Check sheet for the modelled part. Datum: model origin and axes. Units: mm. Round coordinates to 2 decimals unless told otherwise and drop trailing zeros. Order: outer loops, then holes, each group sorted by start corner. A loop starts at its lowest first (then second) coordinate and runs counter-clockwise, first axis right, second up. Notation, with made-up numbers: (64, 84) -> (80, 84) arc R22 ccw to (80, 90) -> close; hole circle Ø7 at (-40, 15.25). An arc over 180 degrees is marked (long way). Answer in a Markdown table with one row per item.
```python
from build123d import *

# Parameters (mm, degrees)
SKETCH_2_R          = 1.5
EXTRUDE_1_DEPTH     = 10
CUT_EXTRUDE_START   = -7.5
SKETCH_3_R          = 1.5
SKETCH_3_R_2        = 1.2
CUT_EXTRUDE_1_DEPTH = 0.6
CHAMFER_1_SIZE      = 0.2


with BuildPart() as part:
    # 草图2 → 凸台-拉伸1 (new body, symmetric)
    with BuildSketch(Plane(origin=(0, 0, 0), x_dir=(0, 0, -1), z_dir=(1, 0, 0))):
        Circle(SKETCH_2_R)
    extrude(amount=EXTRUDE_1_DEPTH, both=True)

    # 草图3 → 切除-拉伸1 (cut)
    with BuildSketch(Plane(origin=(0, 0, 0), x_dir=(0, 0, -1), z_dir=(1, 0, 0)).offset(CUT_EXTRUDE_START)):
        Circle(SKETCH_3_R)
        Circle(SKETCH_3_R_2, mode=Mode.SUBTRACT)
    cut_extrude_1 = extrude(amount=-CUT_EXTRUDE_1_DEPTH, mode=Mode.SUBTRACT)

    # 镜向1: 切除-拉伸1 across plane
    add(cut_extrude_1.mirror(Plane(origin=(0, 0, 0), x_dir=(0, 0, 1), z_dir=(1, 0, 0))), mode=Mode.SUBTRACT)

    # 倒角1
    chamfer_1_edges = [part.edges().sort_by_distance(p)[0] for p in [
        (-10, 0, 1.5),
        (10, 0, 1.5),
    ]]
    chamfer(chamfer_1_edges, length=CHAMFER_1_SIZE)


solid = part.part
```
(1) Section check A-A on x = -2. Record the boundary of the cut face in (y, z), plus the area to 3 significant figures.
Solutions:
| item | result |
|---|---|
| outline | circle Ø3 at (0, 0) |
| area | 7.07 mm^2 |
(2) Scan lines: probe 1 along X at (y, z) = (0.9, 0.85); probe 2 along Z at (x, y) = (5, -0.1); probe 3 along Z at (x, y) = (6.75, 0.9). Record each from-to range of solid material in increasing order. Write a range as from..to.
Solutions:
| item | result |
|---|---|
| probe 1 | -10..-8.1, -7.5..7.5, 8.1..10 |
| probe 2 | -1.5..1.5 |
| probe 3 | -1.2..1.2 |
(3) Draft check along X on faces 1 (the cylindrical face through (-7.8, 1.01, -0.65)), 2 (the flat face through (10, 0, 0)), 3 (the cylindrical face through (7.8, 1.01, -0.65)), 4 (the cylindrical face through (8.96, 0.07, 1.5)). Enter one of: pulls with the +X half, pulls with the -X half, needs draft (parallel to the pull), parting line crosses it, or undercut.
Solutions:
| item | result |
|---|---|
| face 1 | undercut |
| face 2 | pulls with the +X half |
| face 3 | undercut |
| face 4 | needs draft |
